Model file for the job. Use its own axes, mm. Give positions to 0.01 mm unless a question says otherwise; leave off trailing zeros. Write each loop counter-clockwise with the first axis right and the second up, starting at its lowest first coordinate (ties: lowest second). Pieces come first, ordered by that corner, then holes.
```python
from build123d import *

# Parameters (mm, degrees)
F0_R     = 2
F1_DEPTH = 2.55


with BuildPart() as f1:
    # F0 (on Top) → F1 (new body)
    with BuildSketch(Plane.XY):
        with BuildLine():
            ThreePointArc((11.426351, 4.415994), (3.266568, 5.023899), (-0.599572, 12.235318))
            ThreePointArc((-0.599572, 12.235318), (-12.25, 0), (-0.599572, -12.235318))
            ThreePointArc((-0.599572, -12.235318), (3.266568, -5.023899), (11.426351, -4.415994))
            Line((11.426351, -4.415994), (49.83354, -3.499003))
            ThreePointArc((49.83354, -3.499003), (53.25, 0), (49.83354, 3.499003))
            Line((49.83354, 3.499003), (11.426351, 4.415994))
        make_face()
        with Locations((49.75, 0)):
            Circle(F0_R, mode=Mode.SUBTRACT)
    extrude(amount=F1_DEPTH)


solid = f1.part
```
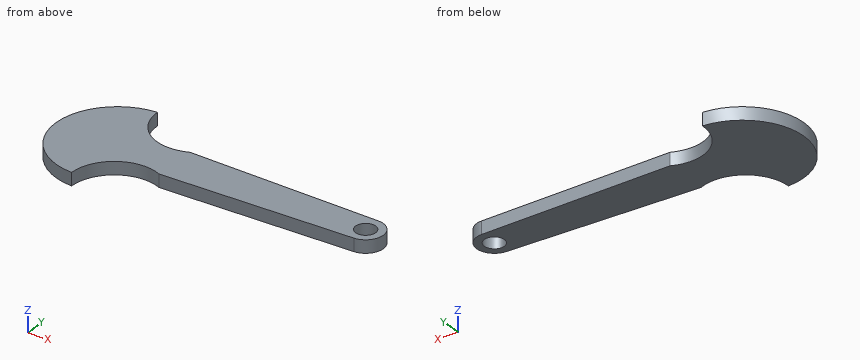
1. Probe probe 1 along Y at (x, z) = (49.75, 0.9); probe 2 along Y at (x, z) = (44, 0.75); probe 3 along Y at (x, z) = (43, 1). List the from-to ranges inside material, lowest first.
Calculated:
probe 1: y = -3.5 to -2, 2 to 3.5
probe 2: y = -3.64 to 3.64
probe 3: y = -3.66 to 3.66
2. Slice it at A-A, the plane y = 0. Write the cut outline in (x, z), and give its area (3 significant figures).
Calculated:
outline: (-12.25, 0) - (47.75, 0) - (47.75, 2.55) - (-12.25, 2.55) - close; (51.75, 0) - (53.25, 0) - (53.25, 2.55) - (51.75, 2.55) - close
area: 157 mm2
3. Slice it at C-C, the plane x = -6. Write the cut outline in (y, z).
Calculated:
outline: (-10.68, 0) - (10.68, 0) - (10.68, 2.55) - (-10.68, 2.55) - close
4. Pin check, flat tips, straight feed: P1, Ø5, axis at x = 49.75, y = 0, coming from the -Z side; P2, Ø6, axis at x = 5.5, y = -7.5, coming from the +Z side. Stop position of each tip, or through.
Calculated:
P1: stops at z = 0
P2: passes through
5. Slice it at D-D, the plane y = -6. Write the cut outline in (x, z), and give its area (3 significant figures).
Calculated:
outline: (-10.68, 0) - (2.03, 0) - (2.03, 2.55) - (-10.68, 2.55) - close
area: 32.4 mm2
6. Slice it at B-B, the plane z = 1.3. Write the cut outline in (x, y), and give its area (3 significant figures).
Calculated:
outline: (-0.6, -12.24) arc R8.5 cw to (11.43, -4.42) - (49.83, -3.5) arc R3.5 ccw to (49.83, 3.5) - (11.43, 4.42) arc R8.5 cw to (-0.6, 12.24) arc R12.25 ccw to start; hole circle Ø4 at (49.75, 0)
area: 652 mm2
